Geometry: see drawing. Coordinates: mm, zero at the bounding-box minimum. A direction names the side the tool comes from. Round coordinates to 2 decimals unless told otherwise and drop trailing zeros. Write each loop counter-clockwise with the first axis right and the second up, starting at its lowest first coordinate (ties: lowest second). Pieces come first, ordered by that corner, then holes.
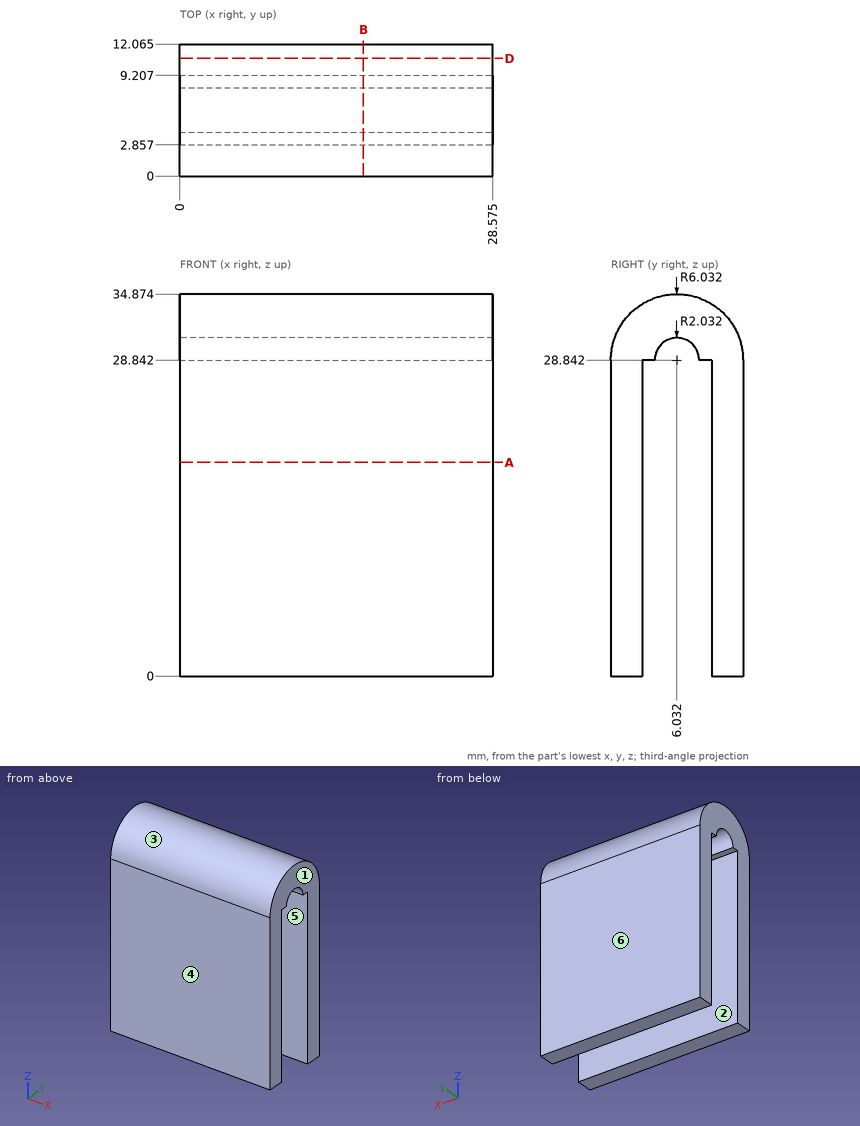
1) Section query D-D on y = 10.75. Return the cut outline in (x, z) (1 decimal).
Taken from the geometry:
outline: (0, 0) - (28.6, 0) - (28.6, 32.6) - (0, 32.6) - close
2) Material intervals for line 1 (Y direction, x = 16.25, z = 7) (1 decimal); line 2 (Z direction, x = 25.5, y = 5.25) (1 decimal); line 3 (Z direction, x = 21.25, y = 11.25), sorted ascending.
Taken from the geometry:
line 1: y = 0 to 2.9, 9.2 to 12.1
line 2: z = 30.7 to 34.8
line 3: z = 0 to 31.87
3) Contact query for flat-ended pins moving along their axis: P1, Ø0.9, axis at x = 15, y = 8.5, coming from the -Z side; P2, Ø1.5, axis at x = 22.5, y = 10, coming from the -Z side; P3, Ø5, axis at x = 20, y = 10.5, coming from the +Z side (1 decimal). Output: stop coordinate, or through.
Taken from the geometry:
P1: stops at z = 28.84
P2: stops at z = 0
P3: stops at z = 34.5
4) Reachability of the marked faces 5 and 6 from +Z, -Z, +X, -X, +Y, -Y: full face, straight path, thin tool, end or side. Return the list, or none.
Taken from the geometry:
face 5: -Z, +X, -X
face 6: +Z, -Z, +X, -X, +Y
5) Section query A-A on z = 19.5. Return the cut outline in (x, y) (1 decimal).
Taken from the geometry:
outline: (0, 0) - (28.6, 0) - (28.6, 2.9) - (0, 2.9) - close; (0, 9.2) - (28.6, 9.2) - (28.6, 12.1) - (0, 12.1) - close
6) Pull-direction query (Y, two-part tool) for the marked faces 1, 2, 3 and 4; classes: released by +Y, released by -Y, zero draft, split by the parting line, or undercut.
Taken from the geometry:
face 1: zero draft
face 2: undercut
face 3: split by the parting line
face 4: released by -Y
7) Section query B-B on x = 16.75. Return the cut outline in (y, z) (1 decimal).
Taken from the geometry:
outline: (0, 0) - (2.9, 0) - (2.9, 28.8) - (4, 28.8) arc R2 cw to (8.1, 28.8) - (9.2, 28.8) - (9.2, 0) - (12.1, 0) - (12.1, 28.8) arc R6 ccw to (0, 28.8) - close
